Work out the finished part from the listing and answer in its coordinate system (mm). Face numbers are marked on the shaded views. A direction names the side the tool comes from. Give positions to 0.01 mm unless a question says otherwise; leave off trailing zeros. Loops run counter-clockwise (first coordinate to the right, second up) from the corner with the lowest first, then second, coordinate; pieces in that order, holes last. Notation, with made-up numbers: (64.5, 75.25) - (76.5, 75.25) arc R31 cw to (76.5, 105.25) - close; hole circle Ø3 at (64.5, 8). An arc over 180 degrees is marked (long way). One line per question, with ' | ' between items. Start each with the question number.
1. Section A-A (x = 0) is taken. Determine the outline of the cut face in (y, z).
2. For a pull along X with two mould halves and no side action, classify the marked faces 1, 2 and 3 as released by +X, released by -X, zero draft, split by the parting line, or undercut.
3. Which of the six approach directions +Z, -Z, +X, -X, +Y, -Y give full straight-line access (tool end or side, diameter ignored) to the marked faces 4 and 5?
4. Each of these flat-tipped pins is pushed along its axis until it touches: pin 1 (1 mm diameter, centred on x = 2, y = 22, fed in from -Z); pin 2 (0.7 mm diameter, centred on x = 0, y = 30.5, fed in from -Z); pin 3 (2 mm diameter, centred on y = 22, z = 1, fed in from +X). Where does it stop, or does it pass through?
5. Section B-B (y = 20) is taken. Determine the outline of the cut face in (x, z), plus the area to 3 significant figures.
6. Find the intervals of material crossed by line 1 (Y direction, x = -0.5, z = 0); line 2 (X direction, y = 20, z = 1.5); line 3 (X direction, y = 12.5, z = 1.25), in increasing order.
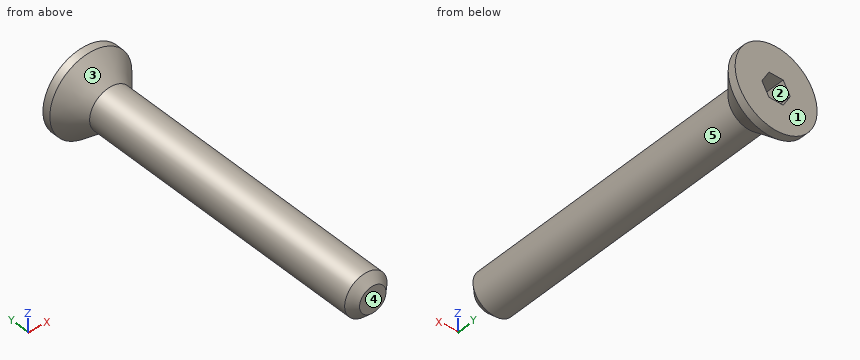
Autodesk Inventor part; units mm, degrees
ref_plane "YZ Plane" through (0, 0, 0) normal (1, 0, 0) x (0, 1, 0)
ref_plane "XZ Plane" through (0, 0, 0) normal (0, 1, 0) x (-1, 0, 0)
ref_plane "XY Plane" through (0, 0, 0) normal (0, 0, 1) x (1, 0, 0)
sketch "Sketch1" plane through (0, 0, 0) normal (0, 0, 1) x (1, 0, 0)
  line L0 (0, 0) -> (3.937, 0)
  line L1 (3.937, 0) -> (3.937, 31.75)
  line L2 (3.937, 31.75) -> (0, 31.75)
  line L3 (0, 31.75) -> (0, 0)
  line L4 (2.032, 28.7965) -> (2.032, 0)
  line L5 (2.032, 28.7965) -> (3.937, 30.988)
  dimension "d0" = 3.937
  dimension "d1" = 31.75
  dimension "d2" = 2.032
  dimension "d3" = 0.762
  dimension "d4" = 41
revolve "Revolution1" add sketch "Sketch1" angle 360 about axis through (0, 31.75, 0) along (0, -1, 0) contours L3 L2 L1 L5 L4 L0
chamfer "Chamfer1" distance 0.762 angle 45 1 edges at (-2.032, 0, 0)
thread "Thread1"
sketch "Sketch2" plane through (0, 31.75, 0) normal (0, 1, 0) x (1, 0, 0)
  line L0 (1.3638, 0) -> (0.6819, -1.1811)
  line L1 (0.6819, -1.1811) -> (-0.6819, -1.1811)
  line L2 (-0.6819, -1.1811) -> (-1.3638, 0)
  line L3 (-1.3638, 0) -> (-0.6819, 1.1811)
  line L4 (-0.6819, 1.1811) -> (0.6819, 1.1811)
  line L5 (0.6819, 1.1811) -> (1.3638, 0)
  point P0 (0, 0)
  point P1 (0, 0)
  point P2 (0, 0)
  dimension "d11" = 2.3622
extrude "Extrusion1" cut sketch "Sketch2" against normal blind 2.286
properties part number "8-32 UNC Flathead Bolt" material "Stainless Steel"
Conclusion:
1) outline: (0, -1.27) - (0.76, -2.03) - (28.8, -2.03) - (30.99, -3.94) - (31.75, -3.94) - (31.75, -1.18) - (29.46, -1.18) - (29.46, 1.18) - (31.75, 1.18) - (31.75, 3.94) - (30.99, 3.94) - (28.8, 2.03) - (0.76, 2.03) - (0, 1.27) - close
2) face 1: zero draft | face 2: undercut | face 3: split by the parting line
3) face 4: +Z, -Z, +X, -X, -Y | face 5: -Y
4) pin 1: z = -1.37 | pin 2: z = -3.82 | pin 3: x = 2.03
5) outline: circle Ø4.06 at (0, 0) | area: 13.0 mm²
6) line 1: 0 to 29.46 | line 2: -1.37 to 1.37 | line 3: -1.6 to 1.6
